Read the model definition and answer for the solid it produces. Units are mm, in the model's axes. Face numbers are marked on the shaded views. A direction names the side the tool comes from. Coordinates: 2 decimals unless noted, no trailing zeros. Order: outer loops, then holes, each group sorted by start corner. A loop starts at its lowest first (then second) coordinate and runs counter-clockwise, first axis right, second up. Notation, with made-up numbers: (-15.75, 65.25) -> (25.25, 65.25) arc R12 cw to (25.25, 69.25) -> close; hole circle Ø8 at (73.25, -27.75). An arc over 180 degrees is marked (long way). Use CSV: the item, a comma, the result in double quotes.
Autodesk Inventor part; units mm, degrees
ref_plane "YZ Plane" through (0, 0, 0) normal (1, 0, 0) x (0, 1, 0)
ref_plane "XZ Plane" through (0, 0, 0) normal (0, 1, 0) x (-1, 0, 0)
ref_plane "XY Plane" through (0, 0, 0) normal (0, 0, 1) x (1, 0, 0)
sketch "Sketch1" plane through (0, 0, 0) normal (0, 0, 1) x (1, 0, 0)
  line L0 (0, 0) -> (18.7452, 0)
  line L1 (18.7452, 0) -> (18.7452, 2.9718)
  line L2 (18.7452, 2.9718) -> (15.6972, 2.9718)
  line L3 (15.6972, 2.9718) -> (15.6972, 1.9558)
  line L4 (15.6972, 1.9558) -> (15.0622, 1.9558)
  line L5 (15.0622, 1.9558) -> (15.0622, 2.9718)
  line L6 (15.0622, 2.9718) -> (13.716, 2.9718)
  line L7 (13.716, 2.9718) -> (13.716, 1.9558)
  line L8 (13.716, 1.9558) -> (10.033, 1.9558)
  line L9 (10.033, 1.9558) -> (10.033, 2.9718)
  line L10 (10.033, 2.9718) -> (8.6868, 2.9718)
  line L11 (8.6868, 2.9718) -> (8.6868, 1.9558)
  line L12 (8.6868, 1.9558) -> (7.5438, 1.9558)
  line L13 (7.5438, 1.9558) -> (7.5438, 2.9718)
  line L14 (7.5438, 2.9718) -> (6.477, 2.9718)
  line L15 (6.477, 2.9718) -> (6.477, 4.445)
  line L16 (6.477, 4.445) -> (5.969, 4.445)
  line L17 (5.969, 4.445) -> (5.969, 1.2785)
  line L18 (0, 0) -> (0, 0.9144)
  line L19 (0, 0.9144) -> (5.969, 1.2785)
  dimension "d0" = 18.7452
  dimension "d1" = 2.9718
  dimension "d2" = 3.048
  dimension "d3" = 1.016
  dimension "d4" = 0.635
  dimension "d5" = 1.3462
  dimension "d6" = 3.683
  dimension "d7" = 1.3462
  dimension "d8" = 1.143
  dimension "d9" = 1.0668
  dimension "d10" = 1.4732
  dimension "d11" = 0.508
  dimension "d12" = 0.9144
revolve "Revolution1" add sketch "Sketch1" angle 360 about axis through (0, 0, 0) along (1, 0, 0)
hole "Hole1" at (0, 0, 0) direction (1, 0, 0) diameter 1.27 depth 12.319 tip angle 118
thread "Thread1"
sketch "Sketch2" plane through (18.7452, 0, 0) normal (1, 0, 0) x (0, 0, -1)
  circle A0 centre (0, 0) radius 2.9718
  line L0 (0, 0) -> (0, 0.635)
  line L1 (0, 0.635) -> (-2.9972, 0.635)
  line L2 (-2.9972, 0.635) -> (2.9718, 0.635)
  line L3 (2.9718, 0.635) -> (2.9718, -0.635)
  line L4 (2.9718, -0.635) -> (-2.9972, -0.635)
  line L5 (-2.9972, -0.635) -> (-2.9972, 0.635)
  dimension "d25" = 0.635
  dimension "d26" = 2.9972
  dimension "d27" = 5.969
  dimension "d28" = 1.27
extrude "Extrusion1" cut sketch "Sketch2" against normal blind 1.5875 contours A0 L4 L1 L2 | L3 L4 A0 | A0 L2 L3 | A0 L4 L5 L1
sketch "Sketch3" plane through (0, 0, 0) normal (0, 0, 1) x (1, 0, 0)
  line L0 (0, 0) -> (12.319, 0)
  dimension "d31" = 12.319
hole "Hole2" at (12.319, 0, 0) direction (0, 0, -1) diameter 0.7874 end through all
properties part number "Carburetor"
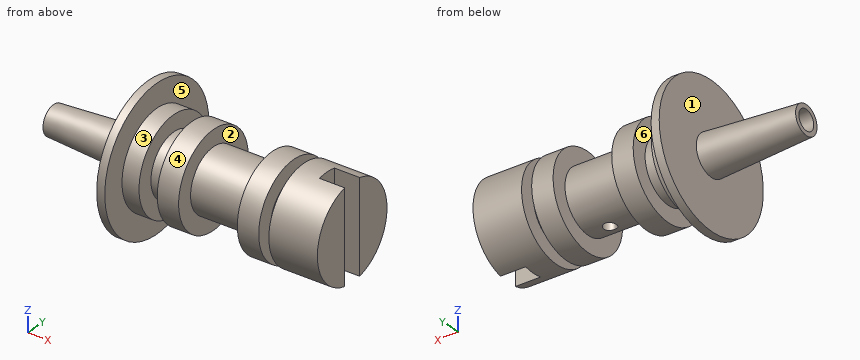
Item 1: A tool of negligible diameter and unlimited length cuts with its end or side. For the marked faces 1, 2 and 3, from which of +Z, -Z, +X, -X, +Y, -Y can it reach the whole face along a straight path? Write none if from no direction.
Return value:
face 1,"-X"
face 2,"none"
face 3,"+X"
Item 2: Find section D-D, the plane z = 3.5. Give the vertices of the cut face in (x, y), then the cut area to 3 significant figures.
Return value:
outline,"(5.97, -2.74) -> (6.48, -2.74) -> (6.48, 2.74) -> (5.97, 2.74) -> close"
area,"2.78 mm^2"
Item 3: Straight lines are drawn through the part: line 1 along X through (y, z) = (-0.5, -2.75); line 2 along X through (y, z) = (-1.75, -1); line 3 along Z through (x, y) = (7.5, 0) (3 decimals). For each, find the intervals that lie inside material, in ascending order.
Return value:
line 1,"x = 5.97 to 7.54, 8.69 to 10.03, 13.72 to 15.06, 15.7 to 17.16"
line 2,"x = 5.97 to 7.54, 8.69 to 10.03, 13.72 to 15.06, 15.7 to 18.75"
line 3,"z = -2.972 to -0.635, 0.635 to 2.972"
Item 4: Find section A-A, the plane y = -2.75. Give the vertices of the cut face in (x, z), then the cut area to 3 significant figures.
Return value:
outline,"(5.97, -3.49) -> (6.48, -3.49) -> (6.48, -1.13) -> (7.54, -1.13) -> (7.54, 1.13) -> (6.48, 1.13) -> (6.48, 3.49) -> (5.97, 3.49) -> close; (8.69, -1.13) -> (10.03, -1.13) -> (10.03, 1.13) -> (8.69, 1.13) -> close; (13.72, -1.13) -> (15.06, -1.13) -> (15.06, 1.13) -> (13.72, 1.13) -> close; (15.7, -1.13) -> (18.75, -1.13) -> (18.75, 1.13) -> (15.7, 1.13) -> close"
area,"18.9 mm^2"
Item 5: Each of these flat-tipped pins is pushed along its axis until it touches: P1, Ø1.8, axis at y = -0.5, z = 0.5, coming from the +X side; P2, Ø1.3, axis at x = 17.5, z = -0.5, coming from the -Y side; P3, Ø1.5, axis at x = 16.5, z = 3, coming from the -Y side; P4, Ø1.1, axis at y = 0, z = 0, coming from the +X side. Where does it stop, or does it pass through?
Return value:
P1,"stops at x = 18.75"
P2,"stops at y = -2.97"
P3,"stops at y = -1.94"
P4,"stops at x = 17.16"
Item 6: Find section C-C, the plane x = 4. Give the vertices of the cut face in (y, z) (3 decimals).
Return value:
outline,"circle Ø2.317 at (0, 0); hole circle Ø1.27 at (0, 0)"
Item 7: The mould has two halves that part along X. Classify the marked faces 4, 5 and 6: +X half, -X half, draft (parallel to the pull), parting line (faces both ways), or undercut.
Return value:
face 4,"draft"
face 5,"+X half"
face 6,"undercut"
